Could you check a few things on this model? Use its own coordinates, in mm. Face numbers are marked on the shaded views. A direction names the side the tool comes from. Coordinates: 2 decimals unless noted, no trailing zeros. Loops run counter-clockwise (first coordinate to the right, second up) from the corner with the lowest first, then second, coordinate; pieces in that order, holes last.
1) If I drill on line 1 along Z through (x, y) = (3, 4.5); line 2 along X through (y, z) = (8, -29); line 3 along Y through (x, z) = (6, -26.05), over which ranges is the centre line in solid material (lowest first)?
2) Thinking about a two-plate mould opening in Z: for the marked faces 3, 4 and 5, which applies, released by +Z, released by -Z, zero draft, split by the parting line, or undercut?
3) For the marked faces 1 and 2, which set-ups out of +Z, -Z, +X, -X, +Y, -Y let a thin tool reach every point of the face, with its end or its side?
4) Imagine slicing it at C-C on x = -12.5. Please give me the cut outline in (y, z).
5) Imagine slicing it at B-B on z = -29. Please give me the cut outline in (x, y), plus the area to 3 significant figures.
6) Imagine slicing it at A-A on x = 0.5. Please give me the cut outline in (y, z).
7) Imagine slicing it at D-D on x = 7.5. Give the number of separate pieces and of enclosed holes in the cut face, plus the area to 3 significant figures.
8) Will these pins go through, and if not, where does the flat tip stop? P1, Ø1.5, axis at y = 5.5, z = -21.5, coming from the +X side; P2, Ø6, axis at x = 4.5, y = 3.5, coming from the +Z side; P3, Ø16, axis at x = -12.5, z = -10, coming from the -Y side; P4, Ø3.5, axis at x = 6, y = 6, coming from the +Z side.
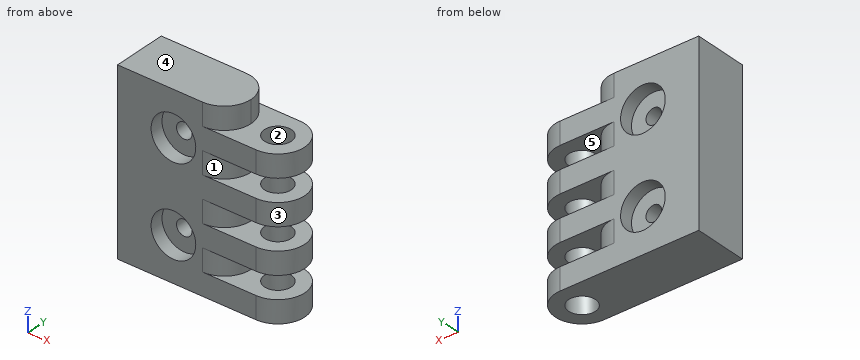
```python
from build123d import *

# Parameters (mm, degrees)
SKETCH1_W           = 25
SKETCH1_H           = 40
BOSS_EXTRUDE1_DEPTH = 12
SKETCH2_R           = 3
BOSS_EXTRUDE2_DEPTH = 40
SKETCH3_W           = 12
SKETCH3_H           = 5
CUT_EXTRUDE1_DEPTH  = 49.672374095
LPATTERN1_COUNT     = 4
LPATTERN1_PITCH     = 10
SKETCH4_R           = 1.75
CUT_EXTRUDE2_DEPTH  = 49.672374095
SKETCH5_R           = 5
CUT_EXTRUDE3_DEPTH  = 3
LPATTERN2_COUNT     = 2
LPATTERN2_PITCH     = 9
FILLET1_R           = 6


with BuildPart() as part:
    # Sketch1 → Boss-Extrude1 (new body)
    with BuildSketch(Plane(origin=(0, 0, 0), x_dir=(1, 0, 0), z_dir=(0, 1, 0))):
        with Locations((-12.5, 20)):
            Rectangle(SKETCH1_W, SKETCH1_H)
    extrude(amount=BOSS_EXTRUDE1_DEPTH)

    # Sketch2 → Boss-Extrude2 (add)
    with BuildSketch(Plane.XY):
        with BuildLine():
            Line((0, 6), (0, 0))
            Line((0, 0), (6, 0))
            ThreePointArc((6, 0), (12, 6), (6, 12))
            Line((6, 12), (0, 12))
            Line((0, 12), (0, 6))
        make_face()
        with Locations((6, 6)):
            Circle(SKETCH2_R, mode=Mode.SUBTRACT)
    extrude(amount=-BOSS_EXTRUDE2_DEPTH)

    # Sketch3 → Cut-Extrude1 (cut, through all)
    with BuildSketch(Plane(origin=(0, 12, 0), x_dir=(1, 0, 0), z_dir=(0, 1, 0))):
        with Locations((6, 32.5)):
            Rectangle(SKETCH3_W, SKETCH3_H)
    cut_extrude1 = extrude(amount=-CUT_EXTRUDE1_DEPTH, mode=Mode.SUBTRACT)

    # LPattern1: Cut-Extrude1 ×4
    with Locations(*[(0, 0, i * LPATTERN1_PITCH) for i in range(1, LPATTERN1_COUNT)]):
        add(cut_extrude1, mode=Mode.SUBTRACT)

    # Sketch4 → Cut-Extrude2 (cut, through all)
    with BuildSketch(Plane(origin=(0, 12, 0), x_dir=(1, 0, 0), z_dir=(0, 1, 0))):
        with Locations(Location((-12.5, 30, 0), (0, 0, 270))):
            Circle(SKETCH4_R)
        with Locations(Location((-12.5, 10, 0), (0, 0, 270))):
            Circle(SKETCH4_R)
    extrude(amount=-CUT_EXTRUDE2_DEPTH, mode=Mode.SUBTRACT)

    # Sketch5 → Cut-Extrude3 (cut)
    with BuildSketch(Plane(origin=(0, 12, 0), x_dir=(1, 0, 0), z_dir=(0, 1, 0))):
        with Locations(Location((-12.5, 30, 0), (0, 0, 270))):
            Circle(SKETCH5_R)
        with Locations(Location((-12.5, 10, 0), (0, 0, 270))):
            Circle(SKETCH5_R)
    cut_extrude3 = extrude(amount=-CUT_EXTRUDE3_DEPTH, mode=Mode.SUBTRACT)

    # LPattern2: Cut-Extrude3 ×2
    with Locations(*[(0, -i * LPATTERN2_PITCH, 0) for i in range(1, LPATTERN2_COUNT)]):
        add(cut_extrude3, mode=Mode.SUBTRACT)

    # Fillet1
    fillet1_edges = [part.edges().sort_by_distance(p)[0] for p in [
        (0, 0, -2.5),
        (0, 12, -2.5),
        (0, 0, -12.5),
        (0, 12, -12.5),
        (0, 0, -22.5),
        (0, 12, -22.5),
        (0, 0, -32.5),
        (0, 12, -32.5),
    ]]
    fillet(fillet1_edges, radius=FILLET1_R - 0.0001)  # a hair under: the kernel refuses the full size


solid = part.part
```
Filled in:
1. line 1: z = -40 to -35, -30 to -25, -20 to -15, -10 to -5
1. line 2: x = -25 to -13.94, -11.06 to 3.76, 8.24 to 11.66
1. line 3: y = 0 to 3, 9 to 12
2. face 3: zero draft
2. face 4: released by +Z
2. face 5: undercut
3. face 1: +X, -Y
3. face 2: +Z, -Z
4. outline: (0, -40) - (12, -40) - (12, -35) - (9, -35) - (9, -31.75) - (3, -31.75) - (3, -35) - (0, -35) - close; (0, -25) - (3, -25) - (3, -28.25) - (9, -28.25) - (9, -25) - (12, -25) - (12, -15) - (9, -15) - (9, -11.75) - (3, -11.75) - (3, -15) - (0, -15) - close; (0, -5) - (3, -5) - (3, -8.25) - (9, -8.25) - (9, -5) - (12, -5) - (12, 0) - (0, 0) - close
5. outline: (-25, 0) - (-17.4, 0) - (-17.4, 3) - (-13.94, 3) - (-13.94, 9) - (-17.4, 9) - (-17.4, 12) - (-25, 12) - close; (-11.06, 3) - (-7.6, 3) - (-7.6, 0) - (6, 0) arc R6 ccw to (6, 12) - (-7.6, 12) - (-7.6, 9) - (-11.06, 9) - close; hole circle Ø6 at (6, 6)
5. area: 324 mm2
6. outline: (0, -40) - (12, -40) - (12, -35) - (0, -35) - close; (0, -30) - (12, -30) - (12, -25) - (0, -25) - close; (0, -20) - (12, -20) - (12, -15) - (0, -15) - close; (0, -10) - (12, -10) - (12, -5) - (0, -5) - close
7. separate pieces: 8
7. enclosed holes: 0
7. area: 128 mm2
8. P1: stops at x = 0
8. P2: stops at z = -5
8. P3: stops at y = 0
8. P4: passes through
